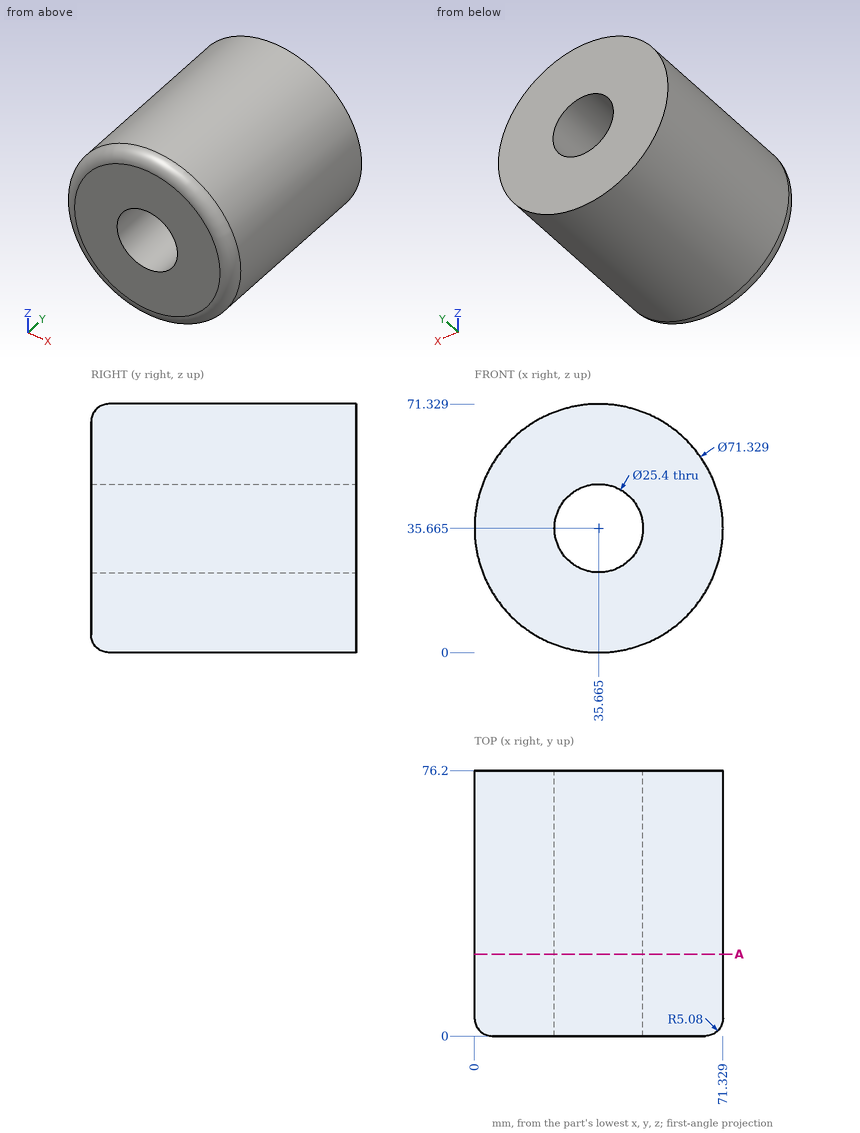
Study the drawing (mm; zero at the part's minimum x, y, z) and answer. Give positions to 0.01 mm unless a question says otherwise; leave off trailing zeros. Write each loop counter-clockwise with the first axis right and the second up, starting at its lowest first coordinate (ties: lowest second). Pieces come first, ordered by that corner, then holes. Notation, with made-up numbers: M -18,87 L 40,87 A29 ccw 40,125 Z; hole C -19.75,73 d9. An arc over 180 degrees is marked long. Put each result on its own line as item: value. Start each with the question number.
1. Each of these flat-tipped pins is pushed along its axis until it touches: pin 1 Ø1 at (y, z) = (54.5, 9.5) entering from +X; pin 2 Ø5 at (x, y) = (11, 63.5) entering from -Z (1 decimal); pin 3 Ø4 at (x, y) = (47.5, 23) entering from -Z. Where does it stop, or does it pass through?
2. Consider line 1 along Z through (x, y) = (43, 61) (1 decimal); line 2 along Z through (x, y) = (41, 51.5); line 3 along X through (y, z) = (29, 45) (1 decimal). Determine where each line is inside the solid, lowest interval first.
3. The part is cut by section A-A, the plane y = 23.5. Give the vertices of the cut face in (x, z) (1 decimal).
Final values:
1. pin 1: stops at x = 60.43
1. pin 2: stops at z = 7.7
1. pin 3: stops at z = 1.38
2. line 1: z = 0.8 to 25.3, 46 to 70.6
2. line 2: z = 0.4 to 24.14, 47.19 to 70.93
2. line 3: x = 1.2 to 27.1, 44.3 to 70.1
3. outline: C 35.7,35.7 d71.3; hole C 35.7,35.7 d25.4
